from build123d import *

# Parameters (mm, degrees)
SKETCH1_R           = 14.605
BOSS_EXTRUDE1_DEPTH = 50.8
SKETCH2_W           = 29.21
SKETCH2_H           = 31.649894197
BOSS_EXTRUDE3_DEPTH = 3.02006
BOSS_EXTRUDE4_DEPTH = 15.24
SKETCH4_W           = 1.524
SKETCH4_H           = 31.858022221
BOSS_EXTRUDE6_DEPTH = 15.875
SKETCH5_W           = 31.726657408
SKETCH5_H           = 31.858022221
SKETCH5_W_2         = 31.767634357
BOSS_EXTRUDE7_DEPTH = 20.066


with BuildPart() as part:
    # Sketch1 → Boss-Extrude1 (new body)
    with BuildSketch(Plane.XY):
        Circle(SKETCH1_R)
    extrude(amount=-BOSS_EXTRUDE1_DEPTH)

    # Sketch2 → Boss-Extrude3 (add)
    with BuildSketch(Plane(origin=(0, 0, -50.8), x_dir=(-1, 0, 0), z_dir=(0, 0, -1))):
        with Locations((0, 15.824947099)):
            Rectangle(SKETCH2_W, SKETCH2_H)
    extrude(amount=-BOSS_EXTRUDE3_DEPTH)

    # Sketch3 → Boss-Extrude4 (add)
    with BuildSketch(Plane(origin=(0, 31.649894197, 0), x_dir=(1, 0, 0), z_dir=(0, 1, 0))):
        Polygon((-14.605, 50.8), (-44.442538052, 50.8), (-44.442538052, 18.941977779), (44.457461948, 18.941977779), (44.457461948, 50.8), align=None)
    extrude(amount=BOSS_EXTRUDE4_DEPTH)

    # Sketch4 → Boss-Extrude6 (add)
    with BuildSketch(Plane(origin=(0, 46.889894197, 0), x_dir=(1, 0, 0), z_dir=(0, 1, 0))):
        with Locations((43.695461948, 34.87098889)):
            Rectangle(SKETCH4_W, SKETCH4_H)
        with Locations((-43.680538052, 34.87098889)):
            Rectangle(SKETCH4_W, SKETCH4_H)
    extrude(amount=BOSS_EXTRUDE6_DEPTH)

    # Sketch5 → Boss-Extrude7 (add)
    with BuildSketch(Plane(origin=(0, 62.764894197, 0), x_dir=(1, 0, 0), z_dir=(0, 1, 0))):
        with Locations((-28.579209348, 34.87098889)):
            Rectangle(SKETCH5_W, SKETCH5_H)
        with Locations((28.573644769, 34.87098889)):
            Rectangle(SKETCH5_W_2, SKETCH5_H)
    extrude(amount=BOSS_EXTRUDE7_DEPTH)


solid = part.part
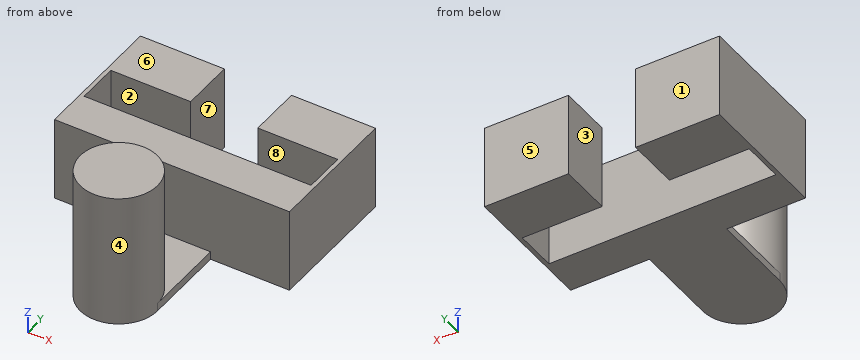
Geometry: final body of the model. Coordinates: model frame, mm. Face numbers are marked on the shaded views. A direction names the side the tool comes from. Give positions to 0.01 mm unless a question says otherwise; leave off trailing zeros. Write each loop counter-clockwise with the first axis right and the second up, starting at its lowest first coordinate (ties: lowest second). Pieces come first, ordered by that corner, then holes. Notation, with made-up numbers: (77.5, 51) -> (95.5, 51) arc R23 ccw to (95.5, 65) -> close; hole circle Ø2 at (67.25, 38). An arc over 180 degrees is marked (long way). Answer as a JSON object with one key per item and string values.
1. Cut plane B-B on z = -46. Output: boundary loops of the cut face in (x, y) (3 decimals).
Ans:
{"outline": "(-44.443, 31.65) -> (44.457, 31.65) -> (44.457, 82.831) -> (12.69, 82.831) -> (12.69, 62.765) -> (42.933, 62.765) -> (42.933, 46.89) -> (-42.919, 46.89) -> (-42.919, 62.765) -> (-12.716, 62.765) -> (-12.716, 82.831) -> (-44.443, 82.831) -> close; circle Ø29.21 at (0, 0)"}
2. Cut plane A-A on x = -16.5. Output: boundary loops of the cut face in (y, z), and give its area (3 significant figures).
Ans:
{"outline": "(31.65, -50.8) -> (46.89, -50.8) -> (46.89, -18.94) -> (31.65, -18.94) -> close; (62.76, -50.8) -> (82.83, -50.8) -> (82.83, -18.94) -> (62.76, -18.94) -> close", "area": "1,120 mm^2"}
3. Mould query, pull axis Y, two halves, no side actions, for the marked faces 1, 2 and 3. Classes: pulls with the +Y half, pulls with the -Y half, needs draft (parallel to the pull), parting line crosses it, or undercut.
Ans:
{"face 1": "pulls with the +Y half", "face 2": "undercut", "face 3": "needs draft"}
4. Access query for the marked faces 4, 5, 6, 7 and 8. Directions: +Z, -Z, +X, -X, +Y, -Y. A direction counts if a zero-diameter tool reaches every point of the face in a straight line with its end or side. Return the directions, or none.
Ans:
{"face 4": "+Z", "face 5": "+Z, -Z, +X, -X, +Y", "face 6": "+Z, +X, -X, +Y", "face 7": "+Z, -Z, +Y", "face 8": "+Z, -Z"}
5. Cut plane C-C on x = 0. Output: boundary loops of the cut face in (y, z) (3 decimals).
Ans:
{"outline": "(-14.605, -50.8) -> (46.89, -50.8) -> (46.89, -18.942) -> (31.65, -18.942) -> (31.65, -47.78) -> (14.605, -47.78) -> (14.605, 0) -> (-14.605, 0) -> close"}
6. Ray query, probe 1 along Y at (x, z) = (-35, -32); probe 2 along X at (y, z) = (66, -31); probe 3 along Z at (x, y) = (-19, 73.5). Return the intervals inside material, ascending. Write a range as from..to.
Ans:
{"probe 1": "y = 31.65..46.89, 62.76..82.83", "probe 2": "x = -44.44..-12.72, 12.69..44.46", "probe 3": "z = -50.8..-18.94"}
7. Cut plane D-D on y = 43.5. Output: boundary loops of the cut face in (x, z).
Ans:
{"outline": "(-44.44, -50.8) -> (44.46, -50.8) -> (44.46, -18.94) -> (-44.44, -18.94) -> close"}
8. Contact query for flat-ended pins moving along their axis: pin 1 (12 mm diameter, centred on y = 25.5, z = -42.5, fed in from +X) (3 decimals); pin 2 (0.9 mm diameter, centred on y = 9, z = -49.5, fed in from -X) (3 decimals); pin 3 (1 mm diameter, centred on y = 16, z = -17, fed in from +X); pin 4 (24 mm diameter, centred on x = -32, z = -28, fed in from -Y). Output: stop coordinate, or through.
Ans:
{"pin 1": "stops at x = 14.605", "pin 2": "stops at x = -14.605", "pin 3": "passes through", "pin 4": "stops at y = 31.65"}
